Check sheet for the modelled part. Datum: model origin and axes. Units: mm. A direction names the side the tool comes from. Round coordinates to 2 decimals unless told otherwise and drop trailing zeros. Loops run counter-clockwise (first coordinate to the right, second up) from the corner with the lowest first, then second, coordinate; pieces in that order, holes last. Notation, with made-up numbers: (-11, 10) - (15, 10) arc R25 ccw to (15, 41) - close; hole circle Ø1 at (1, 33). An arc over 180 degrees is marked (long way). Put each result on its own line as item: value. Start each with the question number.
Item 1: Section check C-C, the plane y = 5. Record the cut outline in (x, z), and give its area (3 significant figures).
Item 2: Section check A-A, the plane z = 0. Record the cut outline in (x, y), and give its area (4 significant figures).
Item 3: Tool access check on faces 4 (the flat face through (-2, 13.5, -2)), 5 (the cylindrical face through (-3.434, 11.774, -1.081)), 6 (the cylindrical face through (-6.2, 5.07, -1.95)). Record the directions out of +Z, -Z, +X, -X, +Y, -Y that give a thin tool (end or side, any length) a straight path to the whole face; none if there is none.
Item 4: Gauge pin test, flat ends, axial feed: pin 1 Ø1 at (x, z) = (-4, -2) entering from -Y; pin 2 Ø5 at (x, y) = (5, 3) entering from +Z; pin 3 Ø3 at (y, z) = (5, 5) entering from +X; pin 4 Ø3 at (y, z) = (5, 0) entering from -X. Record the tip position at first contact, or that the pin passes through.
Item 5: Section check B-B, the plane x = 0. Record the cut outline in (y, z).
Item 6: Section check D-D, the plane y = 19. Record the cut outline in (x, z).
Item 7: Material ranges on line 1 along Y through (x, z) = (-3.5, 0); line 2 along Y through (x, z) = (-2.5, 0); line 3 along Y through (x, z) = (-1.5, 2.5), recorded low to high.
Item 8: Draft check along Y on faces 1 (the flat face through (0, 0, 0)), 2 (the cylindrical face through (-0.09, 3.29, 0.38)), 3 (the flat face through (-3, 10, 3)). Enter one of: pulls with the +Y half, pulls with the -Y half, needs draft (parallel to the pull), parting line crosses it, or undercut.
from build123d import *

# Parameters (mm, degrees)
CUT_EXTRUDE1_DEPTH      = 27.636441204
CUT_EXTRUDE1_DEPTH_BACK = 27.636441204
SKETCH2_R               = 1.75


with BuildPart() as part:
    # Sketch1 → Revolve1 (revolve)
    with BuildSketch(Plane.XY):
        Polygon((0, 0), (-6.5, 0), (-6.5, 10), (-3.6, 10), (-3.6, 13.5), (-2.6, 13.5), (-2.6, 17.5), (-3.6, 17.5), (-3.6, 25), (0, 25), align=None)
    revolve(axis=Axis((0, 25, 0), (0, -1, 0)))

    # Sketch2 → Cut-Extrude1 (cut, two sides: drawn at the far end of the back side and taken through both)
    with BuildSketch(Plane(origin=(0, 0, 0), x_dir=(0, 0, -1), z_dir=(1, 0, 0)).offset(-CUT_EXTRUDE1_DEPTH_BACK)):
        with Locations((0, 5)):
            Circle(SKETCH2_R)
    extrude(amount=CUT_EXTRUDE1_DEPTH + CUT_EXTRUDE1_DEPTH_BACK, mode=Mode.SUBTRACT)


solid = part.part
Check result:
1. outline: (-6.26, -1.75) arc R6.5 ccw to (6.26, -1.75) - close; (-6.26, 1.75) - (6.26, 1.75) arc R6.5 ccw to start
1. area: 87.8 mm²
2. outline: (-6.5, 0) - (6.5, 0) - (6.5, 3.25) - (-6.5, 3.25) - close; (-6.5, 6.75) - (6.5, 6.75) - (6.5, 10) - (3.6, 10) - (3.6, 13.5) - (2.6, 13.5) - (2.6, 17.5) - (3.6, 17.5) - (3.6, 25) - (-3.6, 25) - (-3.6, 17.5) - (-2.6, 17.5) - (-2.6, 13.5) - (-3.6, 13.5) - (-3.6, 10) - (-6.5, 10) - close
2. area: 184.5 mm²
3. face 4: none
3. face 5: +Y
3. face 6: +Y, -Y
4. pin 1: y = 0
4. pin 2: z = 6
4. pin 3: x = 5.48
4. pin 4: through
5. outline: (0, -6.5) - (10, -6.5) - (10, -3.6) - (13.5, -3.6) - (13.5, -2.6) - (17.5, -2.6) - (17.5, -3.6) - (25, -3.6) - (25, 3.6) - (17.5, 3.6) - (17.5, 2.6) - (13.5, 2.6) - (13.5, 3.6) - (10, 3.6) - (10, 6.5) - (0, 6.5) - close; hole circle Ø3.5 at (5, 0)
6. outline: circle Ø7.2 at (0, 0)
7. line 1: 0 to 3.25, 6.75 to 13.5, 17.5 to 25
7. line 2: 0 to 3.25, 6.75 to 25
7. line 3: 0 to 13.5, 17.5 to 25
8. face 1: pulls with the -Y half
8. face 2: undercut
8. face 3: pulls with the +Y half
